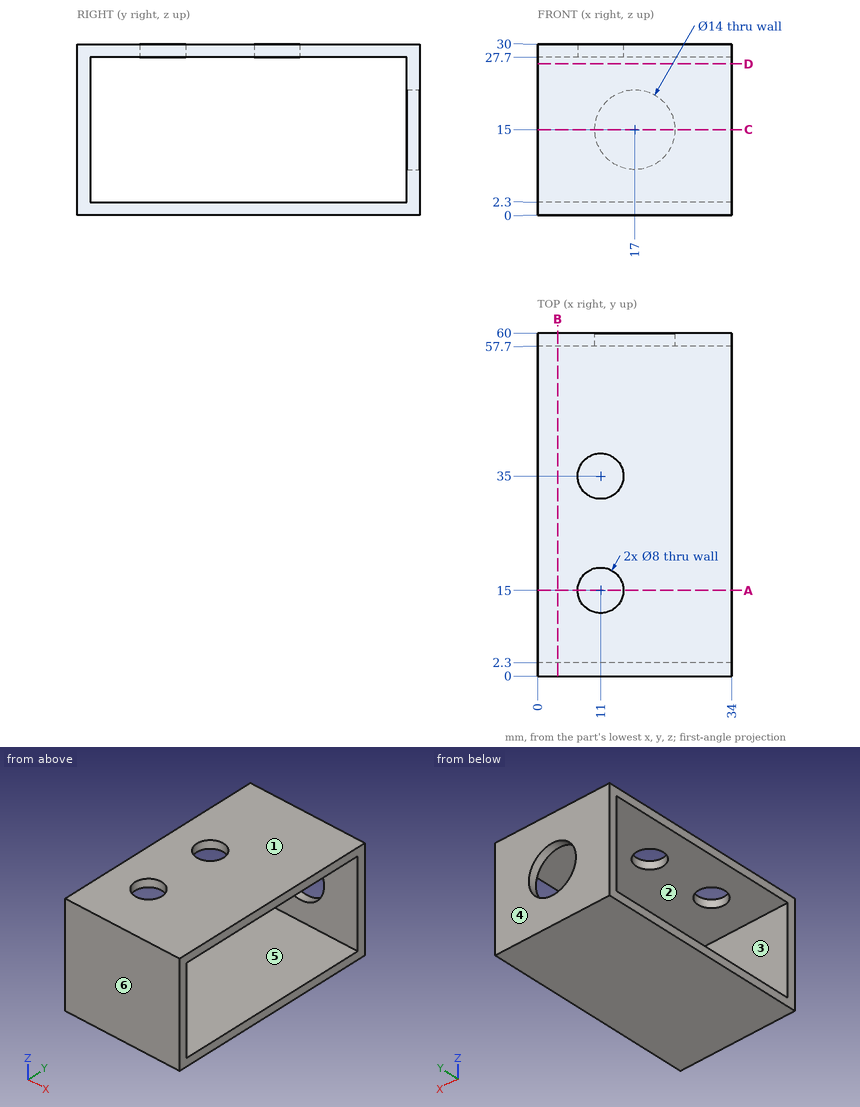
Answer from the drawing. Dimensions are ordinates in mm from the lowest x, y and z of the part. A direction names the side the tool comes from. Give positions to 0.01 mm unless a question says otherwise; leave off trailing zeros. Write each loop counter-clockwise with the first axis right and the second up, starting at its lowest first coordinate (ties: lowest second). Pieces come first, ordered by that corner, then holes.
1) For a pull along Z with two mould halves and no side action, classify the marked faces 1, 2, 3 and 4 as pulls with the +Z half, pulls with the -Z half, needs draft (parallel to the pull), parting line crosses it, or undercut.
2) Section D-D (z = 26.5) is taken. Write down the section's boundary in (x, y), and give its area (3 significant figures).
3) Section B-B (x = 3.5) is taken. Write down the section's boundary in (y, z), and give its area (3 significant figures).
4) Given P1, Ø6.5, axis at x = 11, y = 15, coming from the +Z side; P2, Ø1, axis at x = 21, z = 19.5, coming from the +Y side, each flat-ended and moving along its own axis, determine where each tip first touches the part or whether it passes through.
5) A tool of negligible diameter and unlimited length cuts with its end or side. For the marked faces 5 and 6, from which of +Z, -Z, +X, -X, +Y, -Y can it reach the whole face along a straight path? Write none if from no direction.
6) Find the intervals of material crossed by L1, parallel to Y at x = 11, z = 28.45; L2, parallel to Y at x = 13, z = 5.75; L3, parallel to Z at x = 13, y = 30, in increasing order.
7) Section A-A (y = 15) is taken. Write down the section's boundary in (x, z).
8) Section C-C (z = 15) is taken. Write down the section's boundary in (x, y).
Response:
1. face 1: pulls with the +Z half
1. face 2: undercut
1. face 3: undercut
1. face 4: needs draft
2. outline: (0, 0) - (34, 0) - (34, 2.3) - (0, 2.3) - close; (0, 57.7) - (34, 57.7) - (34, 60) - (0, 60) - close
2. area: 156 mm2
3. outline: (0, 0) - (60, 0) - (60, 30) - (0, 30) - close; hole (2.3, 2.3) - (57.7, 2.3) - (57.7, 27.7) - (2.3, 27.7) - close
3. area: 393 mm2
4. P1: stops at z = 2.3
4. P2: stops at y = 2.3
5. face 5: +X, -X
5. face 6: +Z, -Z, +X, -X, -Y
6. L1: y = 0 to 11, 19 to 31, 39 to 60
6. L2: y = 0 to 2.3, 57.7 to 60
6. L3: z = 0 to 2.3, 27.7 to 30
7. outline: (0, 0) - (34, 0) - (34, 2.3) - (0, 2.3) - close; (0, 27.7) - (7, 27.7) - (7, 30) - (0, 30) - close; (15, 27.7) - (34, 27.7) - (34, 30) - (15, 30) - close
8. outline: (0, 0) - (34, 0) - (34, 2.3) - (0, 2.3) - close; (0, 57.7) - (10, 57.7) - (10, 60) - (0, 60) - close; (24, 57.7) - (34, 57.7) - (34, 60) - (24, 60) - close
